```python
from build123d import *

# Parameters (mm, degrees)
SKETCH2_R          = 1.5
CUT_EXTRUDE1_DEPTH = 33.595091655


with BuildPart() as part:
    # Sketch1 → Revolve1 (revolve)
    with BuildSketch(Plane.XY, mode=Mode.PRIVATE) as revolve1_sk:
        Polygon((-10.5, 20.2), (-10.5, 14.2), (-8.5, 14.2), (-8.5, 12.2), (-10.5, 12.2), (-10.5, 0), (-20, 0), (-20, 4), (-12.5, 4), (-12.5, 20.2), align=None)
    revolve(revolve1_sk.sketch.rotate(Axis((0, 0, 0), (0, 1, 0)), 270), axis=Axis((0, 0, 0), (0, 1, 0)))

    # Sketch2 → Cut-Extrude1 (cut, through all)
    with BuildSketch(Plane(origin=(0, 4, 0), x_dir=(1, 0, 0), z_dir=(0, 1, 0))):
        with Locations(Location((0, 15.5, 0), (0, 0, 270))):
            Circle(SKETCH2_R)
        with Locations(Location((15.5, 0, 0), (0, 0, 270))):
            Circle(SKETCH2_R)
        with Locations(Location((0, -15.5, 0), (0, 0, 270))):
            Circle(SKETCH2_R)
        with Locations(Location((-15.5, 0, 0), (0, 0, 270))):
            Circle(SKETCH2_R)
    extrude(amount=-CUT_EXTRUDE1_DEPTH, mode=Mode.SUBTRACT)


solid = part.part
```
Geometry: final body of the model. Coordinates: model frame, mm. A direction names the side the tool comes from. Round coordinates to 2 decimals unless told otherwise and drop trailing zeros. Write each loop counter-clockwise with the first axis right and the second up, starting at its lowest first coordinate (ties: lowest second). Pieces come first, ordered by that corner, then holes.
Item 1: Section query A-A (x = 0). Return loops of the section in (y, z), plus the area to 3 significant figures.
Item 2: Material intervals for L1, parallel to X at y = 2.85, z = 0; L2, parallel to X at y = 17.55, z = 0; L3, parallel to X at y = 13.05, z = 0, sorted ascending.
Item 3: Section query D-D (z = -6). Return loops of the section in (x, y).
Item 4: Section query B-B (z = 0). Return loops of the section in (x, y).
Item 5: Mould query, pull axis Z, two halves, no side actions, for faces 1 (the face through (-3.755, 12.213, -11.923)), 2 (the face through (-3.2, 17.2, -10)), 3 (the face through (9, 0, 9)). Classes: +Z half, -Z half, draft (parallel to the pull), parting line (faces both ways), or undercut.
Item 6: Set-up query: faces 4 (the face through (-8.428, 13.186, 1.107)), 5 (the face through (0, 12.2, 9)), 6 (the face through (0, 14.2, -9)). Return all of +Z, -Z, +X, -X, +Y, -Y with unobstructed straight access to the full face (end or side cutting, diameter ignored); none if empty.
Item 7: Section query C-C (x = -15.5). Return loops of the section in (y, z).
Item 8: Pin query (flat end, axial travel): P1, Ø2, axis at y = 5.5, z = 7.5, coming from the -X side; P2, Ø3.5, axis at x = 15.5, z = 0, coming from the +Y side; P3, Ø1, axis at y = 13.5, z = 7.5, coming from the -X side. Return the tip coordinate at first contact, or that it passes through.
Completed:
1. outline: (0, -20) - (4, -20) - (4, -17) - (0, -17) - close; (0, -14) - (4, -14) - (4, -12.5) - (20.2, -12.5) - (20.2, -10.5) - (14.2, -10.5) - (14.2, -8.5) - (12.2, -8.5) - (12.2, -10.5) - (0, -10.5) - close; (0, 10.5) - (12.2, 10.5) - (12.2, 8.5) - (14.2, 8.5) - (14.2, 10.5) - (20.2, 10.5) - (20.2, 12.5) - (4, 12.5) - (4, 14) - (0, 14) - close; (0, 17) - (4, 17) - (4, 20) - (0, 20) - close
1. area: 125 mm2
2. L1: x = -20 to -17, -14 to -10.5, 10.5 to 14, 17 to 20
2. L2: x = -12.5 to -10.5, 10.5 to 12.5
2. L3: x = -12.5 to -8.5, 8.5 to 12.5
3. outline: (-19.08, 0) - (-8.62, 0) - (-8.62, 12.2) - (-6.02, 12.2) - (-6.02, 14.2) - (-8.62, 14.2) - (-8.62, 20.2) - (-10.97, 20.2) - (-10.97, 4) - (-19.08, 4) - close; (6.02, 12.2) - (8.62, 12.2) - (8.62, 0) - (19.08, 0) - (19.08, 4) - (10.97, 4) - (10.97, 20.2) - (8.62, 20.2) - (8.62, 14.2) - (6.02, 14.2) - close
4. outline: (-20, 0) - (-17, 0) - (-17, 4) - (-20, 4) - close; (-14, 0) - (-10.5, 0) - (-10.5, 12.2) - (-8.5, 12.2) - (-8.5, 14.2) - (-10.5, 14.2) - (-10.5, 20.2) - (-12.5, 20.2) - (-12.5, 4) - (-14, 4) - close; (8.5, 12.2) - (10.5, 12.2) - (10.5, 0) - (14, 0) - (14, 4) - (12.5, 4) - (12.5, 20.2) - (10.5, 20.2) - (10.5, 14.2) - (8.5, 14.2) - close; (17, 0) - (20, 0) - (20, 4) - (17, 4) - close
5. face 1: parting line
5. face 2: undercut
5. face 3: draft
6. face 4: +Y, -Y
6. face 5: -Y
6. face 6: +Y
7. outline: (0, -12.64) - (4, -12.64) - (4, -1.5) - (0, -1.5) - close; (0, 1.5) - (4, 1.5) - (4, 12.64) - (0, 12.64) - close
8. P1: stops at x = -10.68
8. P2: stops at y = 4
8. P3: stops at x = -10.36
